from build123d import *

# Parameters (mm, degrees)
BOSS_EXTRUDE1_START = -5
SKETCH1_R           = 13.717927936
BOSS_EXTRUDE1_DEPTH = 5
SKETCH2_W           = 6.9
SKETCH2_H           = 6.9
BOSS_EXTRUDE2_DEPTH = 20


with BuildPart() as part:
    # Sketch1 → Boss-Extrude1 (new body)
    with BuildSketch(Plane.XY.offset(BOSS_EXTRUDE1_START)):
        with Locations((1.150128538, -20.08136278)):
            Circle(SKETCH1_R)
    extrude(amount=-BOSS_EXTRUDE1_DEPTH)

    # Sketch2 → Boss-Extrude2 (add)
    with BuildSketch(Plane(origin=(0, 0, -10), x_dir=(-1, 0, 0), z_dir=(0, 0, -1))):
        with Locations((0, -20)):
            Rectangle(SKETCH2_W, SKETCH2_H)
    extrude(amount=BOSS_EXTRUDE2_DEPTH)


solid = part.part
Here's how the part is built. I have some questions about the finished solid (model axes, mm). A direction names the side the tool comes from. Coordinates: 2 decimals unless noted, no trailing zeros. Order: outer loops, then holes, each group sorted by start corner. A loop starts at its lowest first (then second) coordinate and runs counter-clockwise, first axis right, second up. Notation, with made-up numbers: (75.5, 82.5) -> (83.5, 82.5) arc R18 ccw to (83.5, 87.5) -> close; hole circle Ø6 at (87, 84). An arc over 180 degrees is marked (long way). Answer in a Markdown table with one row per item.
(1) On a 3-axis mill with a long thin cutter (end or side, diameter ignored), from which of +Z, -Z, +X, -X, +Y, -Y can I reach the whole of each face in a straight line? I mean faces 1 (the face through (0, -23.45, -20)), 2 (the face through (-3.45, -20, -20)), 3 (the face through (0, -16.55, -20)), 4 (the face through (3.45, -20, -20)). Say none if no direction works.
Answer key:
| item | result |
|---|---|
| face 1 | -Z, +X, -X, -Y |
| face 2 | -Z, -X, +Y, -Y |
| face 3 | -Z, +X, -X, +Y |
| face 4 | -Z, +X, +Y, -Y |
(2) Will these pins go through, and if not, where does the flat tip stop? pin 1 Ø7.5 at (y, z) = (-21.5, -16) entering from +X; pin 2 Ø8 at (x, z) = (-4.5, -27) entering from -Y; pin 3 Ø7.5 at (y, z) = (-21, -25) entering from -X; pin 4 Ø1 at (x, z) = (5.5, -15) entering from -Y.
Answer key:
| item | result |
|---|---|
| pin 1 | x = 3.45 |
| pin 2 | y = -23.45 |
| pin 3 | x = -3.45 |
| pin 4 | through |
(3) I want a section at B-B on z = -15.25. List the corners of the cut face in (x, y) for me.
Answer key:
| item | result |
|---|---|
| outline | (-3.45, -23.45) -> (3.45, -23.45) -> (3.45, -16.55) -> (-3.45, -16.55) -> close |
(4) I want a section at A-A on x = -1. List the corners of the cut face in (y, z) for me.
Answer key:
| item | result |
|---|---|
| outline | (-33.63, -10) -> (-23.45, -10) -> (-23.45, -30) -> (-16.55, -30) -> (-16.55, -10) -> (-6.53, -10) -> (-6.53, -5) -> (-33.63, -5) -> close |
(5) I want a section at C-C on y = -28.75. List the corners of the cut face in (x, z) for me, then the cut area to 3 significant figures.
Answer key:
| item | result |
|---|---|
| outline | (-9.48, -10) -> (11.78, -10) -> (11.78, -5) -> (-9.48, -5) -> close |
| area | 106 mm^2 |
(6) Please list where these lines run through material, in increasing order: probe 1 along Z at (x, y) = (2.25, -31); probe 2 along Y at (x, z) = (0, -21.75); probe 3 along X at (y, z) = (-20, -7).
Answer key:
| item | result |
|---|---|
| probe 1 | -10 to -5 |
| probe 2 | -23.45 to -16.55 |
| probe 3 | -12.57 to 14.87 |
